Here's how the part is built. I have some questions about the finished solid (model axes, mm). Face numbers are marked on the shaded views. A direction names the side the tool comes from. Give positions to 0.01 mm unless a question says otherwise; leave off trailing zeros. Write each loop counter-clockwise with the first axis right and the second up, starting at its lowest first coordinate (ties: lowest second). Pieces come first, ordered by that corner, then holes. Notation, with made-up numbers: (33, 20.5) - (67, 20.5) arc R32 cw to (67, 53.5) - close; hole circle Ø10 at (85.5, 89.5). An arc over 180 degrees is marked (long way). Use one line per item in the form item = value. Start each with the question number.
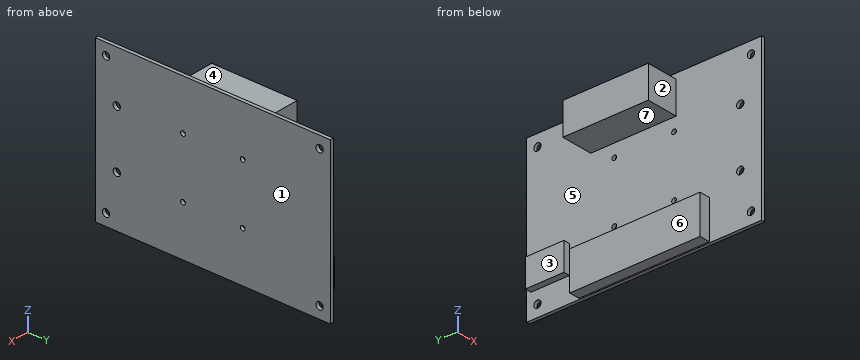
from build123d import *

# Parameters (mm, degrees)
BOARD_START                         = -30
BOARD_SKETCH_W                      = 75
BOARD_SKETCH_H                      = 110
BOARD_SKETCH_R                      = 1.7
BOARD_SKETCH_R_2                    = 1.1
BOARD_DEPTH                         = 1.6
TEENSY_START                        = -31.6
TEENSY_4_1_SKETCH_W                 = 18
TEENSY_4_1_SKETCH_H                 = 61
TEENSY_4_1_DEPTH                    = 5
BAROMETER_START                     = -31.6
BAROMETER_BMP388_BOARD_EST_SKETCH_W = 13
BAROMETER_BMP388_BOARD_EST_SKETCH_H = 18
BAROMETER_BMP388_BOARD_EST_DEPTH    = 3
VENT_START                          = -31.6
VENT_BACKUP_SKETCH_W                = 15
VENT_BACKUP_SKETCH_H                = 40
VENT_BACKUP_DEPTH                   = 15


with BuildPart() as part:
    # Board Sketch → Board (new body)
    with BuildSketch(Plane(origin=(0, 0, 0), x_dir=(0, 0, -1), z_dir=(1, 0, 0)).offset(BOARD_START)):
        Rectangle(BOARD_SKETCH_W, BOARD_SKETCH_H)
        with Locations((32, -50)):
            Circle(BOARD_SKETCH_R, mode=Mode.SUBTRACT)
        with Locations((-32, -50)):
            Circle(BOARD_SKETCH_R, mode=Mode.SUBTRACT)
        with Locations((32, 50)):
            Circle(BOARD_SKETCH_R, mode=Mode.SUBTRACT)
        with Locations((-32, 50)):
            Circle(BOARD_SKETCH_R, mode=Mode.SUBTRACT)
        with Locations((13.5, -45)):
            Circle(BOARD_SKETCH_R, mode=Mode.SUBTRACT)
        with Locations((-13.5, -45)):
            Circle(BOARD_SKETCH_R, mode=Mode.SUBTRACT)
        with Locations((14, -14)):
            Circle(BOARD_SKETCH_R_2, mode=Mode.SUBTRACT)
        with Locations((-14, -14)):
            Circle(BOARD_SKETCH_R_2, mode=Mode.SUBTRACT)
        with Locations((14, 14)):
            Circle(BOARD_SKETCH_R_2, mode=Mode.SUBTRACT)
        with Locations((-14, 14)):
            Circle(BOARD_SKETCH_R_2, mode=Mode.SUBTRACT)
    extrude(amount=-BOARD_DEPTH)

    # Teensy 4.1 Sketch → Teensy 4.1 (add)
    with BuildSketch(Plane(origin=(0, 0, 0), x_dir=(0, 0, -1), z_dir=(1, 0, 0)).offset(TEENSY_START)):
        with Locations((28, 0)):
            Rectangle(TEENSY_4_1_SKETCH_W, TEENSY_4_1_SKETCH_H)
    extrude(amount=-TEENSY_4_1_DEPTH)

    # Barometer BMP388 board [est] Sketch → Barometer BMP388 board [est] (add)
    with BuildSketch(Plane(origin=(0, 0, 0), x_dir=(0, 0, -1), z_dir=(1, 0, 0)).offset(BAROMETER_START)):
        with Locations((19.5, 44)):
            Rectangle(BAROMETER_BMP388_BOARD_EST_SKETCH_W, BAROMETER_BMP388_BOARD_EST_SKETCH_H)
    extrude(amount=-BAROMETER_BMP388_BOARD_EST_DEPTH)

    # Vent backup Sketch → Vent backup (add)
    with BuildSketch(Plane(origin=(0, 0, 0), x_dir=(0, 0, -1), z_dir=(1, 0, 0)).offset(VENT_START)):
        with Locations((-27.5, 5)):
            Rectangle(VENT_BACKUP_SKETCH_W, VENT_BACKUP_SKETCH_H)
    extrude(amount=-VENT_BACKUP_DEPTH)


solid = part.part
1. I want a section at C-C, the plane y = 40. List the corners of the cut face in (x, z) for me, then the cut area to 3 significant figures.
2. I want a section at D-D, the plane z = 14. List the corners of the cut face in (x, y) for me, then the cut area to 3 significant figures.
3. For the marked faces 1, 2 and 3, which set-ups out of +Z, -Z, +X, -X, +Y, -Y let a thin tool reach every point of the face, with its end or its side?
4. Please list where these lines run through material, in increasing order: line 1 (Y direction, x = -31, z = 32); line 2 (Y direction, x = -30.6, z = -13.5); line 3 (Z direction, x = -34, y = 6).
5. For P1, Ø4, axis at x = -36, y = -7.5, coming from the -Z side; P2, Ø5.5, axis at y = -50, z = -32, coming from the -X side; P3, Ø2.5, axis at y = 50, z = 32, coming from the +X side; P4, Ø0.9, axis at x = -33.5, y = 44, coming from the -Z side, each with a flat end and sliding along its axis, tell me the tip position at first contact or that it passes through.
6. I want a section at A-A, the plane y = -45. List the corners of the cut face in (x, z) for me.
7. We'd pull the mould along Z, two halves only. Please class the marked faces 4, 5, 6 and 7: pulls with the +Z half, pulls with the -Z half, needs draft (parallel to the pull), parting line crosses it, or undercut.
8. I want a section at B-B, the plane z = -23.5. List the corners of the cut face in (x, y) for me.
Result sheet:
q1.outline = (-34.6, -26) - (-31.6, -26) - (-31.6, -37.5) - (-30, -37.5) - (-30, 37.5) - (-31.6, 37.5) - (-31.6, -13) - (-34.6, -13) - close
q1.area = 159 mm2
q2.outline = (-31.6, -55) - (-30, -55) - (-30, -46.62) - (-31.6, -46.62) - close; (-31.6, -43.38) - (-30, -43.38) - (-30, -15.1) - (-31.6, -15.1) - close; (-31.6, -12.9) - (-30, -12.9) - (-30, 12.9) - (-31.6, 12.9) - close; (-31.6, 15.1) - (-30, 15.1) - (-30, 55) - (-31.6, 55) - close
q2.area = 164 mm2
q3.face_1 = +Z, -Z, +X, +Y, -Y
q3.face_2 = +Z, -X, -Y
q3.face_3 = +Z, -Z, -X, +Y
q4.line_1 = -55 to -51.7, -48.3 to 48.3, 51.7 to 55
q4.line_2 = -55 to -46.7, -43.3 to -14.98, -13.02 to 13.02, 14.98 to 55
q4.line_3 = -37 to -19, 20 to 35
q5.P1 = -37
q5.P2 = -31.6
q5.P3 = through
q5.P4 = -26
q6.outline = (-31.6, -37.5) - (-30, -37.5) - (-30, -15.2) - (-31.6, -15.2) - close; (-31.6, -11.8) - (-30, -11.8) - (-30, 11.8) - (-31.6, 11.8) - close; (-31.6, 15.2) - (-30, 15.2) - (-30, 37.5) - (-31.6, 37.5) - close
q7.face_4 = pulls with the +Z half
q7.face_5 = undercut
q7.face_6 = needs draft
q7.face_7 = undercut
q8.outline = (-36.6, -30.5) - (-31.6, -30.5) - (-31.6, -55) - (-30, -55) - (-30, 55) - (-31.6, 55) - (-31.6, 53) - (-34.6, 53) - (-34.6, 35) - (-31.6, 35) - (-31.6, 30.5) - (-36.6, 30.5) - close
